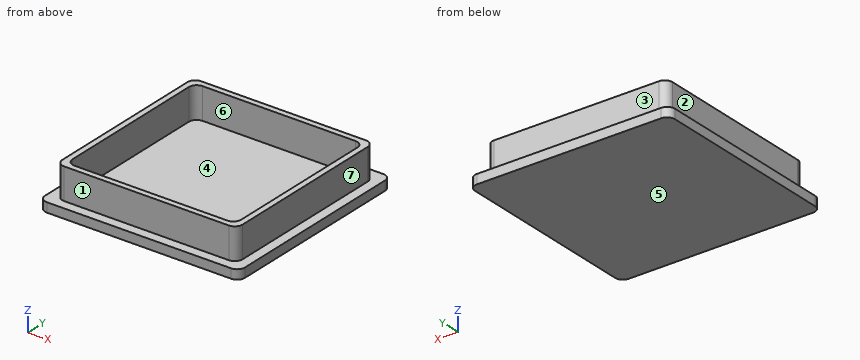
from build123d import *

# Parameters (mm, degrees)
F0_W     = 25.5
F0_H     = 25.5
F1_DEPTH = 1.2
F2_W     = 23
F2_H     = 23
F2_W_2   = 21.5
F2_H_2   = 21.5
F3_DEPTH = 4
F4_R     = 1
F5_R     = 1


with BuildPart() as f1:
    # F0 (on Top) → F1 (new body)
    with BuildSketch(Plane.XY):
        Rectangle(F0_W, F0_H)
    extrude(amount=F1_DEPTH)

    # F2 (on face) → F3 (join)
    with BuildSketch(Plane.XY.offset(1.2)):
        Rectangle(F2_W, F2_H)
        Rectangle(F2_W_2, F2_H_2, mode=Mode.SUBTRACT)
    extrude(amount=F3_DEPTH)

    # F4
    f4_edges = [f1.edges().sort_by_distance(p)[0] for p in [
        (-10.75, 10.75, 3.2),
        (10.75, 10.75, 3.2),
        (10.75, -10.75, 3.2),
        (-10.75, -10.75, 3.2),
    ]]
    fillet(f4_edges, radius=F4_R)

    # F5
    f5_edges = [f1.edges().sort_by_distance(p)[0] for p in [
        (11.5, 11.5, 3.2),
        (11.5, -11.5, 3.2),
        (-11.5, 11.5, 3.2),
        (-11.5, -11.5, 3.2),
        (-12.75, 12.75, 0.6),
        (12.75, 12.75, 0.6),
        (12.75, -12.75, 0.6),
        (-12.75, -12.75, 0.6),
    ]]
    fillet(f5_edges, radius=F5_R)


solid = f1.part
Verification items for the finished model (mm, model axes). Face numbers are marked on the shaded views. A direction names the side the tool comes from. Give positions to 0.01 mm unless a question says otherwise; leave off trailing zeros. Loops run counter-clockwise (first coordinate to the right, second up) from the corner with the lowest first, then second, coordinate; pieces in that order, holes last. Notation, with made-up numbers: (26.25, 34) - (41.25, 34) arc R26 ccw to (41.25, 50) - close; hole circle Ø9 at (74, 58). An arc over 180 degrees is marked (long way). Write each question's results on one line, items separated by ' | '.
1) Sectioned sample at A-A on x = 4.5. Record the boundary of the cut face in (y, z).
Solution:
outline: (-12.75, 0) - (12.75, 0) - (12.75, 1.2) - (11.5, 1.2) - (11.5, 5.2) - (10.75, 5.2) - (10.75, 1.2) - (-10.75, 1.2) - (-10.75, 5.2) - (-11.5, 5.2) - (-11.5, 1.2) - (-12.75, 1.2) - close
2) Mould release check, pull along X, two halves, no side actions. Record for the marked faces 5, 6 and 7: pulls with the +X half, pulls with the -X half, needs draft (parallel to the pull), parting line crosses it, or undercut.
Solution:
face 5: needs draft | face 6: undercut | face 7: pulls with the +X half
3) Tool access check on the marked faces 1, 2, 3 and 4. Record the directions out of +Z, -Z, +X, -X, +Y, -Y that give a thin tool (end or side, any length) a straight path to the whole face; none if there is none.
Solution:
face 1: +Z, +X, -X, -Y | face 2: +Z, -X, +Y, -Y | face 3: +Z, +X, -X, +Y | face 4: +Z
4) Material ranges on L1, parallel to Y at x = 5, z = 4.85; L2, parallel to Z at x = -2.5, y = -4, recorded low to high. Write a range as from..to.
Solution:
L1: -11.5..-10.75, 10.75..11.5 | L2: 0..1.2
5) Sectioned sample at B-B on z = 2.4. Record the boundary of the cut face in (x, y), plus the area to 4 significant figures.
Solution:
outline: (-11.5, -10.5) arc R1 ccw to (-10.5, -11.5) - (10.5, -11.5) arc R1 ccw to (11.5, -10.5) - (11.5, 10.5) arc R1 ccw to (10.5, 11.5) - (-10.5, 11.5) arc R1 ccw to (-11.5, 10.5) - close; hole (-10.75, -9.75) arc R1 ccw to (-9.75, -10.75) - (9.75, -10.75) arc R1 ccw to (10.75, -9.75) - (10.75, 9.75) arc R1 ccw to (9.75, 10.75) - (-9.75, 10.75) arc R1 ccw to (-10.75, 9.75) - close | area: 66.75 mm2
6) Depth check by flat-ended pin: P1, Ø2, axis at y = -4, z = 4, coming from the -X side; P2, Ø2, axis at x = 1, z = 2.5, coming from the +Y side; P3, Ø4, axis at x = 2, y = -3.5, coming from the +Z side. Enter the tip coordinate at first touch or a pass-through.
Solution:
P1: x = -11.5 | P2: y = 11.5 | P3: z = 1.2
